Check sheet for the modelled part. Datum: model origin and axes. Units: mm. Give positions to 0.01 mm unless a question says otherwise; leave off trailing zeros. Write each loop counter-clockwise with the first axis right and the second up, starting at its lowest first coordinate (ties: lowest second). Pieces come first, ordered by that corner, then holes. Notation, with made-up numbers: M 75,78.5 L 108,78.5 A19 ccw 108,108.5 Z; hole C -10,-36.5 d5. An arc over 180 degrees is marked long. Write item = value, one per line. Start each with the question number.
1) Gauge pin test, flat ends, axial feed: pin 1 (1.4 mm diameter, centred on x = 47.5, y = -19, fed in from +Z); pin 2 (6 mm diameter, centred on x = -30, z = -154.5, fed in from +Y); pin 3 (1.4 mm diameter, centred on x = 46.5, y = -19, fed in from -Z). Record the tip position at first contact, or that the pin passes through.
2) Sectioned sample at A-A, the plane z = -158.5. Record the cut outline in (x, y), then the cut area to 3 significant figures.
3) Draft check along X on faces 1 (the face through (48, -19, -188)), 2 (the face through (2.544, -0.592, -3.536)). Enter one of: pulls with the +X half, pulls with the -X half, needs draft (parallel to the pull), parting line crosses it, or undercut.
4) Scan lines: L1, parallel to Y at x = -30.5, z = -13; L2, parallel to Y at x = -6, z = -154. Record each from-to range of solid material in increasing order.
5) Sectioned sample at B-B, the plane y = 5.5. Record the cut outline in (x, z).
6) Sectioned sample at C-C, the plane x = 39.5. Record the cut outline in (y, z).
Autodesk Inventor part; units mm, degrees
ref_plane "YZ Plane" through (0, 0, 0) normal (1, 0, 0) x (0, 1, 0)
ref_plane "XZ Plane" through (0, 0, 0) normal (0, 1, 0) x (-1, 0, 0)
ref_plane "XY Plane" through (0, 0, 0) normal (0, 0, 1) x (1, 0, 0)
sketch "スケッチ1" plane through (0, 0, 0) normal (0, 0, 1) x (1, 0, 0)
  line L0 (-53.8577, -21) -> (53.8577, -21)
  line L1 (53.8577, -21) -> (53.8577, -19.5)
  line L2 (53.8577, -19.5) -> (45.423, -16.1743)
  line L3 (45.423, -16.1743) -> (44.506, -18.5)
  line L4 (44.506, -18.5) -> (-49.7747, 18.6743)
  line L5 (-49.7747, 18.6743) -> (-48.8577, 21)
  line L6 (-48.8577, 21) -> (-53.8577, 21)
  line L7 (-53.8577, 21) -> (-53.8577, -21)
  line L8 (-42.0411, 10.2503) -> (14.7433, -12.1394)
  arc A0 (14.0097, -16) -> (14.7433, -12.1394) centre (14.0097, -14) ccw
  line L9 (14.0097, -16) -> (-42.7747, -16)
  arc A1 (-44.7747, -14) -> (-42.7747, -16) centre (-42.7747, -14) ccw
  line L10 (-44.7747, -14) -> (-44.7747, 8.3897)
  arc A2 (-42.0411, 10.2503) -> (-44.7747, 8.3897) centre (-42.7747, 8.3897) ccw
  line L11 (-48.8577, 21) -> (45.423, -16.1743)
  point P0 (0, 0)
extrude "押し出し1" add sketch "スケッチ1" against normal blind 198 contours L11 L3 L4 L5
ref_plane "作業平面1" through (0, 0, -10) normal (0, 0, 1) x (1, 0, 0)
sketch "スケッチ2" plane through (0, 0, 0) normal (0, 0, 1) x (1, 0, 0)
  line L0 (-53.8577, -21) -> (53.8577, -21)
  line L1 (53.8577, -21) -> (53.8577, -19.5)
  line L2 (53.8577, -19.5) -> (45.423, -16.1743)
  line L3 (45.423, -16.1743) -> (44.506, -18.5)
  line L4 (44.506, -18.5) -> (-49.7747, 18.6743)
  line L5 (-49.7747, 18.6743) -> (-48.8577, 21)
  line L6 (-48.8577, 21) -> (-53.8577, 21)
  line L7 (-53.8577, 21) -> (-53.8577, -21)
  line L8 (-42.0411, 10.2503) -> (14.7433, -12.1394)
  arc A0 (14.0097, -16) -> (14.7433, -12.1394) centre (14.0097, -14) ccw
  line L9 (14.0097, -16) -> (-42.7747, -16)
  arc A1 (-44.7747, -14) -> (-42.7747, -16) centre (-42.7747, -14) ccw
  line L10 (-44.7747, -14) -> (-44.7747, 8.3897)
  arc A2 (-42.0411, 10.2503) -> (-44.7747, 8.3897) centre (-42.7747, 8.3897) ccw
  line L11 (45.423, -16.1743) -> (44.506, -18.5)
  line L12 (44.506, -18.5) -> (50.8464, -21)
  line L13 (50.8464, -21) -> (51.7634, -18.6743)
  line L14 (51.7634, -18.6743) -> (45.423, -16.1743)
  point P0 (0, 0)
extrude "押し出し2" add sketch "スケッチ2" against normal blind 178 from surface at -10 contours L12 L3 L2 L13
sketch "スケッチ3" plane through (-48.8577, 21, 0) normal (0.3668, 0.9303, 0) x (0.9303, -0.3668, 0)
  circle A0 centre (56.0638, 5) radius 1.5
  circle A1 centre (25.5443, 5) radius 1.5
  circle A2 centre (25.5443, 193) radius 1.5
  circle A3 centre (56.0638, 193) radius 1.5
  point P0 (53.1551, 0)
extrude "押し出し3" cut sketch "スケッチ3" against normal blind 2.5
properties part number "Slope_Riner" material "木材 (カエデ材)"
Data:
q1.pin_1 = -10
q1.pin_2 = 14.75
q1.pin_3 = -188
q2.outline = M -49.77,18.67 L 44.51,-18.5 L 50.85,-21 L 51.76,-18.67 L 45.42,-16.17 L -48.86,21 Z
q2.area = 270 mm2
q3.face_1 = needs draft
q3.face_2 = undercut
q4.L1 = 11.07 to 13.76
q4.L2 = 1.41 to 4.1
q5.outline = M -16.36,-198 L -9.55,-198 L -9.55,0 L -16.36,0 Z
q6.outline = M -16.53,-198 L -13.84,-198 L -13.84,0 L -16.53,0 Z
